Work out the finished part from the listing and answer in its coordinate system (mm). A direction names the side the tool comes from. Round coordinates to 2 decimals unless told otherwise and drop trailing zeros. Order: outer loops, then holes, each group sorted by start corner. A loop starts at its lowest first (then second) coordinate and runs counter-clockwise, first axis right, second up. Notation, with made-up numbers: (13.5, 2.5) - (65.5, 2.5) arc R20 ccw to (65.5, 31.5) - close; hole circle Ø6 at (62.5, 37). An arc over 180 degrees is marked (long way). Use CSV: the item, a comma, the result in double quotes.
from build123d import *

# Parameters (mm, degrees)
SKETCH2_W           = 35
SKETCH2_H           = 54.7
SKETCH2_R           = 1.35
SKETCH2_W_2         = 21
SKETCH2_H_2         = 40.7
BOSS_EXTRUDE1_DEPTH = 30
CUT_EXTRUDE2_REACH  = 46.207
BORDES_SERVO_R      = 1.5
ALTURA_TORRES_DEPTH = 46.65665
BOSS_EXTRUDE3_START = 46.65665
SKETCH5_3_W         = 6.975
SKETCH5_3_H         = 6
BOSS_EXTRUDE3_DEPTH = 2
CHAMFER1_SIZE       = 6.975
BOSS_EXTRUDE4_START = 46.65665
SKETCH5_4_R         = 1.6
BOSS_EXTRUDE4_DEPTH = 4
BORDES_EXT_R        = 5


with BuildPart() as part:
    # Sketch2 → Boss-Extrude1 (new body)
    with BuildSketch(Plane(origin=(0, 0, 0), x_dir=(1, 0, 0), z_dir=(0, 1, 0))):
        Rectangle(SKETCH2_W, SKETCH2_H)
        with Locations(Location((-5, 24.75, 0), (0, 0, 270))):
            Circle(SKETCH2_R, mode=Mode.SUBTRACT)
        with Locations(Location((5, 24.75, 0), (0, 0, 90))):
            Circle(SKETCH2_R, mode=Mode.SUBTRACT)
        with Locations(Location((-5, -24.75, 0), (0, 0, 90))):
            Circle(SKETCH2_R, mode=Mode.SUBTRACT)
        with Locations(Location((5, -24.75, 0), (0, 0, 270))):
            Circle(SKETCH2_R, mode=Mode.SUBTRACT)
        Rectangle(SKETCH2_W_2, SKETCH2_H_2, mode=Mode.SUBTRACT)
    extrude(amount=-BOSS_EXTRUDE1_DEPTH)

    # Sketch4 → Cut-Extrude2 (cut, up to next)
    with BuildSketch(Plane(origin=(0, 0, 0), x_dir=(1, 0, 0), z_dir=(0, 1, 0)), mode=Mode.PRIVATE) as cut_extrude2_sk1:
        with BuildLine():
            Line((-3.199984377, -25.852499805), (-3.181265624, -27.35))
            Line((-3.181265624, -27.35), (3.181265624, -27.35))
            Line((3.181265624, -27.35), (3.199984377, -25.852499805))
            ThreePointArc((3.199984377, -25.852499805), (3.329330747, -23.093556632), (3.647756443, -20.35))
            Line((3.647756443, -20.35), (-3.647756443, -20.35))
            ThreePointArc((-3.647756443, -20.35), (-3.329330747, -23.093556632), (-3.199984377, -25.852499805))
        make_face()
    cut_extrude2_tool1 = extrude(cut_extrude2_sk1.sketch, amount=-CUT_EXTRUDE2_REACH, mode=Mode.PRIVATE) & part.part
    add(cut_extrude2_tool1.solids().sort_by_distance((0, 0, 23.771279))[0], mode=Mode.SUBTRACT)

    # Bordes_Servo
    bordes_servo_edges = [part.edges().sort_by_distance(p)[0] for p in [
        (10.5, -30, 0),
        (-7.073878222, -30, 20.35),
        (-10.5, -30, 0),
        (0, -30, -20.35),
        (7.073878222, -30, 20.35),
    ]]
    fillet(bordes_servo_edges, radius=BORDES_SERVO_R)

    # Sketch5 → Altura torres (add)
    with BuildSketch(Plane.XZ.offset(30)):
        Polygon((-12, 21.025), (-17.5, 21.025), (-17.5, -1.025), (-12, -1.025), (-12, 4.975), (-12, 15.025), align=None)
        Polygon((12, 4.975), (12, -1.025), (17.5, -1.025), (17.5, 21.025), (12, 21.025), (12, 15.025), align=None)
    extrude(amount=ALTURA_TORRES_DEPTH)

    # Sketch5<3> → Boss-Extrude3 (add)
    with BuildSketch(Plane.XZ.offset(30).offset(BOSS_EXTRUDE3_START)):
        with Locations((-8.5125, 18.025)):
            Rectangle(SKETCH5_3_W, SKETCH5_3_H)
        with Locations((-8.5125, 1.975)):
            Rectangle(SKETCH5_3_W, SKETCH5_3_H)
        with Locations((8.5125, 1.975)):
            Rectangle(SKETCH5_3_W, SKETCH5_3_H)
        with Locations((8.5125, 18.025)):
            Rectangle(SKETCH5_3_W, SKETCH5_3_H)
    extrude(amount=-BOSS_EXTRUDE3_DEPTH)

    # Chamfer1
    chamfer1_edges = [part.edges().sort_by_distance(p)[0] for p in [
        (12, -74.65665, 18.025),
        (12, -74.65665, 1.975),
        (-12, -74.65665, 18.025),
        (-12, -74.65665, 1.975),
    ]]
    chamfer(chamfer1_edges, length=CHAMFER1_SIZE - 0.0001)  # a hair under: the kernel refuses the full size

    # Sketch5<4> → Boss-Extrude4 (add)
    with BuildSketch(Plane.XZ.offset(30).offset(BOSS_EXTRUDE4_START)):
        with Locations(Location((8.025, 1.975, 0), (0, 0, 270))):
            Circle(SKETCH5_4_R)
        with Locations(Location((-8.025, 1.975, 0), (0, 0, 270))):
            Circle(SKETCH5_4_R)
        with Locations(Location((-8.025, 18.025, 0), (0, 0, 270))):
            Circle(SKETCH5_4_R)
        with Locations(Location((8.025, 18.025, 0), (0, 0, 270))):
            Circle(SKETCH5_4_R)
    extrude(amount=BOSS_EXTRUDE4_DEPTH)

    # Bordes_Ext
    bordes_ext_edges = [part.edges().sort_by_distance(p)[0] for p in [
        (17.5, -76.65665, 10),
        (17.5, -15, -27.35),
        (17.5, -15, 27.35),
        (-17.5, -15, 27.35),
        (-17.5, -15, -27.35),
        (-17.5, -76.65665, 10),
    ]]
    fillet(bordes_ext_edges, radius=BORDES_EXT_R)


solid = part.part
(1) Find the intervals of material crossed by L1, parallel to X at y = -17.75, z = 24.75; L2, parallel to X at y = -8.5, z = -24.75; L3, parallel to X at y = -12, z = -24, in increasing order. Write a range as from..to.
Findings below:
L1,"x = -16.89..-6.35, -3.65..-3.23, 3.23..3.65, 6.35..16.89"
L2,"x = -16.89..-6.35, -3.65..3.65, 6.35..16.89"
L3,"x = -17.22..-6.12, -3.88..3.88, 6.12..17.22"
(2) Find section C-C (y = -7.5). Determine the outline of the cut face in (x, z), and give its area (3 significant figures).
Findings below:
outline,"(-17.5, -22.35) arc R5 ccw to (-12.5, -27.35) - (12.5, -27.35) arc R5 ccw to (17.5, -22.35) - (17.5, 22.35) arc R5 ccw to (12.5, 27.35) - (3.18, 27.35) - (3.2, 25.85) arc R40.21 ccw to (3.65, 20.35) - (10.5, 20.35) - (10.5, -20.35) - (-10.5, -20.35) - (-10.5, 20.35) - (-3.65, 20.35) arc R40.21 ccw to (-3.2, 25.85) - (-3.18, 27.35) - (-12.5, 27.35) arc R5 ccw to (-17.5, 22.35) - close; hole circle Ø2.7 at (-5, -24.75); hole circle Ø2.7 at (-5, 24.75); hole circle Ø2.7 at (5, -24.75); hole circle Ø2.7 at (5, 24.75)"
area,"969 mm²"
(3) Find section A-A (z = -16). Determine the outline of the cut face in (x, y).
Findings below:
outline,"(-17.5, -30) - (-12, -30) arc R1.5 ccw to (-10.5, -28.5) - (-10.5, 0) - (-17.5, 0) - close; (10.5, -28.5) arc R1.5 ccw to (12, -30) - (17.5, -30) - (17.5, 0) - (10.5, 0) - close"
(4) The mould has two halves that part along Z. Classify faces 4 (the cylindrical face through (-6.44, -78.63, 2.18)), 5 (the flat face through (14, -53, 21.025)), 6 (the flat face through (-14, -53, -1.025)), 7 (the flat face through (-8, -80.657, 18)): released by +Z, released by -Z, zero draft, split by the parting line, or undercut.
Findings below:
face 4,"undercut"
face 5,"released by +Z"
face 6,"released by -Z"
face 7,"zero draft"
(5) Find section B-B (y = -61). Determine the outline of the cut face in (x, z) (3 decimals).
Findings below:
outline,"(-17.5, -1.025) - (-12, -1.025) - (-12, 21.025) - (-17.5, 21.025) - close; (12, -1.025) - (17.5, -1.025) - (17.5, 21.025) - (12, 21.025) - close"
(6) For faces 1 (the flat face through (14, -53, -1.025)), 2 (the flat face through (-5.025, -76, 2)), 3 (the flat face through (-7, -14, 20.35)), determine the directions among +Z, -Z, +X, -X, +Y, -Y from which every point of the face is accessible in a straight line to the end or side of a thin tool.
Findings below:
face 1,"-Z, +X, -X, -Y"
face 2,"+Z, -Z, +Y, -Y"
face 3,"+Y"
(7) Each of these flat-tipped pins is pushed along its axis until it touches: pin 1 (10 mm diameter, centred on x = -14, y = -56, fed in from -Z) (3 decimals); pin 2 (1 mm diameter, centred on x = 13.5, z = -13.5, fed in from -Y); pin 3 (2 mm diameter, centred on x = -8, y = -73, fed in from +Z) (3 decimals). Where does it stop, or does it pass through?
Findings below:
pin 1,"stops at z = -1.025"
pin 2,"stops at y = -30"
pin 3,"stops at z = 21.025"
(8) Find section D-D (z = 11.5). Determine the outline of the cut face in (x, y).
Findings below:
outline,"(-17.5, -71.66) arc R5 ccw to (-12.5, -76.66) - (-12, -76.66) - (-12, -30) arc R1.5 ccw to (-10.5, -28.5) - (-10.5, 0) - (-17.5, 0) - close; (10.5, -28.5) arc R1.5 ccw to (12, -30) - (12, -76.66) - (12.5, -76.66) arc R5 ccw to (17.5, -71.66) - (17.5, 0) - (10.5, 0) - close"
